from build123d import *

# Parameters (mm, degrees)
F0_W      = 73
F0_H      = 120
F1_DEPTH  = 50
F3_DEPTH  = 80
F5_DEPTH  = 80
F6_R      = 3.5
F7_DEPTH  = 5
F8_W      = 40
F8_H      = 50
F9_DEPTH  = 73
F10_R     = 5
F11_DEPTH = 80


with BuildPart() as f1:
    # F0 (on Front) → F1 (new body)
    with BuildSketch(Plane.XZ):
        Rectangle(F0_W, F0_H)
    extrude(amount=F1_DEPTH)

    # F2 (on face) → F3 (cut)
    with BuildSketch(Plane(origin=(-36.5, 0, 0), x_dir=(0, -1, 0), z_dir=(-1, 0, 0))):
        with BuildLine():
            ThreePointArc((14.9997541366, 19.5), (34.4997541366, 0), (14.9997541366, -19.5))
            ThreePointArc((14.9997541366, -19.5), (11.4997541366, -23), (14.9997541366, -26.5))
            ThreePointArc((14.9997541366, -26.5), (41.4997541366, 0), (14.9997541366, 26.5))
            ThreePointArc((14.9997541366, 26.5), (11.4997541366, 23), (14.9997541366, 19.5))
        make_face()
    extrude(amount=-F3_DEPTH, mode=Mode.SUBTRACT)

    # F4 (on face) → F5 (cut)
    with BuildSketch(Plane(origin=(-36.5, 0, 0), x_dir=(0, -1, 0), z_dir=(-1, 0, 0))):
        Polygon((50, 60), (0, 60), (50, 25), align=None)
        Polygon((50, -25), (0, -60), (50, -60), align=None)
    extrude(amount=-F5_DEPTH, mode=Mode.SUBTRACT)

    # F6 (on face) → F7 (cut)
    with BuildSketch(Plane(origin=(0, 0, 0), x_dir=(-1, 0, 0), z_dir=(0, 1, 0))):
        with Locations((-21.5, 40)):
            Circle(F6_R)
        with Locations((21.5, 40)):
            Circle(F6_R)
        with Locations((-21.5, -40)):
            Circle(F6_R)
        with Locations((21.5, -40)):
            Circle(F6_R)
    extrude(amount=-F7_DEPTH, mode=Mode.SUBTRACT)

    # F8 (on face) → F9 (join)
    with BuildSketch(Plane(origin=(-36.5, 0, 0), x_dir=(0, -1, 0), z_dir=(-1, 0, 0))):
        with Locations((70, 0)):
            Rectangle(F8_W, F8_H)
    extrude(amount=-F9_DEPTH)

    # F10 (on face) → F11 (cut)
    with BuildSketch(Plane.XY.offset(25)):
        with Locations((0, -70)):
            Circle(F10_R)
    extrude(amount=-F11_DEPTH, mode=Mode.SUBTRACT)


solid = f1.part
Read the model definition and answer for the solid it produces. Units are mm, in the model's axes. A direction names the side the tool comes from. Round coordinates to 2 decimals unless told otherwise and drop trailing zeros. Write each loop counter-clockwise with the first axis right and the second up, starting at its lowest first coordinate (ties: lowest second). Pieces come first, ordered by that corner, then holes. Notation, with made-up numbers: (32, -8) - (58, -8) arc R26 ccw to (58, 28) - close; hole circle Ø11 at (-23, 88). An arc over 180 degrees is marked (long way). One line per question, with ' | ' between items. Start each with the question number.
1. Section D-D (x = -21.5) is taken. Determine the outline of the cut face in (y, z), and give its area (3 significant figures).
2. Section C-C (y = -70) is taken. Determine the outline of the cut face in (x, z).
3. Section B-B (z = 0) is taken. Determine the outline of the cut face in (x, y), and give its area (3 significant figures).
4. Find the intervals of material crossed by probe 1 along Z at (x, y) = (-22, -17.5); probe 2 along Z at (x, y) = (-21, -1); probe 3 along Y at (x, z) = (0, -12), in increasing order. Write a range as [from, to].
5. Each of these flat-tipped pins is pushed along its axis until it touches: pin 1 (3.5 mm diameter, centred on x = 21.5, z = -40, fed in from +Y); pin 2 (11 mm diameter, centred on x = 21.5, z = -40, fed in from -Y); pin 3 (3 mm diameter, centred on x = -27.5, z = -47, fed in from -Y). Where does it stop, or does it pass through?
6. Section A-A (x = 0) is taken. Determine the outline of the cut face in (y, z).
7. For a pull along Y with two mould halves and no side action, classify faces 6 (the face through (-21, -5, -40)), 7 (the face through (-0.511, -34.495, 0.429)), 8 (the face through (21.96, -2.46, -36.53)), 9 (the face through (-0.511, -24.65, 42.745)) as +Y half, -Y half, draft (parallel to the pull), parting line (faces both ways), or undercut.
8. For faces 1 (the face through (-9, -70, -25)), 2 (the face through (-1, -90, 0)), 3 (the face through (-0.511, -41.493, -0.583)), 4 (the face through (-21, -5, 40)), 5 (the face through (36.5, -34, 1)), determine the directions among +Z, -Z, +X, -X, +Y, -Y from which every point of the face is accessible in a straight line to the end or side of a thin tool.
Filled in:
1) outline: (-90, -25) - (-50, -25) - (0, -60) - (0, -43.5) - (-5, -43.5) - (-5, -36.5) - (0, -36.5) - (0, 36.5) - (-5, 36.5) - (-5, 43.5) - (0, 43.5) - (0, 60) - (-50, 25) - (-90, 25) - close; hole (-15, -26.5) arc R3.5 ccw to (-15, -19.5) arc R19.5 cw to (-15, 19.5) arc R3.5 ccw to (-15, 26.5) arc R26.5 ccw to start | area: 5,640 mm²
2) outline: (-36.5, -25) - (-5, -25) - (-5, 25) - (-36.5, 25) - close; (5, -25) - (36.5, -25) - (36.5, 25) - (5, 25) - close
3) outline: (-36.5, -90) - (36.5, -90) - (36.5, -41.5) - (-36.5, -41.5) - close; (-36.5, -34.5) - (36.5, -34.5) - (36.5, 0) - (-36.5, 0) - close; hole circle Ø10 at (0, -70) | area: 5,980 mm²
4) probe 1: [-47.75, -26.38], [-19.34, 19.34], [26.38, 47.75] | probe 2: [-59.3, -43.46], [-36.54, 36.54], [43.46, 59.3] | probe 3: [-90, -75], [-65, -38.63], [-30.37, 0]
5) pin 1: y = -5 | pin 2: y = -36.43 | pin 3: y = -20.71
6) outline: (-90, -25) - (-75, -25) - (-75, 25) - (-90, 25) - close; (-65, -25) - (-50, -25) - (0, -60) - (0, 60) - (-50, 25) - (-65, 25) - close; hole (-15, -26.5) arc R3.5 ccw to (-15, -19.5) arc R19.5 cw to (-15, 19.5) arc R3.5 ccw to (-15, 26.5) arc R26.5 ccw to start
7) face 6: +Y half | face 7: undercut | face 8: draft | face 9: -Y half
8) face 1: -Z, +X, -X, -Y | face 2: +Z, -Z, +X, -X, -Y | face 3: +X, -X | face 4: +Y | face 5: +Z, -Z, +X, +Y, -Y
